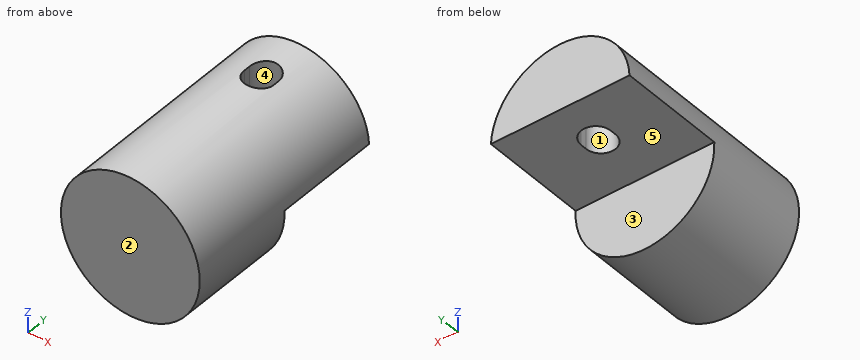
```python
from build123d import *

# Parameters (mm, degrees)
SKETCH1_R               = 9.75
BOSS_EXTRUDE1_DEPTH     = 30
CUT_EXTRUDE1_DEPTH      = 0.5
CUT_EXTRUDE1_DEPTH_BACK = 30
SKETCH3_W               = 19.5
SKETCH3_H               = 15
CUT_EXTRUDE2_DEPTH      = 30


with BuildPart() as part:
    # Sketch1 → Boss-Extrude1 (new body)
    with BuildSketch(Plane(origin=(0, 0, 0), x_dir=(1, 0, 0), z_dir=(0, 1, 0))):
        with Locations(Location((0, 0, 0), (0, 0, 270))):
            Circle(SKETCH1_R)
    extrude(amount=BOSS_EXTRUDE1_DEPTH)

    # Sketch3 → Cut-Extrude1 (cut, two sides: drawn at the far end of the back side and taken through both)
    with BuildSketch(Plane.XY.offset(-CUT_EXTRUDE1_DEPTH_BACK)):
        with Locations((0, 22.5)):
            Rectangle(SKETCH3_W, SKETCH3_H)
    extrude(amount=CUT_EXTRUDE1_DEPTH + CUT_EXTRUDE1_DEPTH_BACK, mode=Mode.SUBTRACT)

    # Sketch4 → Cut-Extrude2 (cut)
    with BuildSketch(Plane(origin=(0, 0, 0.5), x_dir=(-1, 0, 0), z_dir=(0, 0, -1))):
        with BuildLine():
            Line((2.06, 23.683843632), (2.06, 22.803843632))
            ThreePointArc((2.06, 22.803843632), (0, 20.743843632), (-2.06, 22.803843632))
            Line((-2.06, 22.803843632), (-2.06, 23.683843632))
            ThreePointArc((-2.06, 23.683843632), (0, 25.743843632), (2.06, 23.683843632))
        make_face()
    extrude(amount=-CUT_EXTRUDE2_DEPTH, mode=Mode.SUBTRACT)


solid = part.part
```
The listing builds one solid part. Answer for the finished solid, in the listing's coordinates (mm). Face numbers are marked on the shaded views. A direction names the side the tool comes from. Coordinates: 2 decimals unless noted, no trailing zeros. Write each loop counter-clockwise with the first axis right and the second up, starting at its lowest first coordinate (ties: lowest second). Pieces come first, ordered by that corner, then holes. Notation, with made-up numbers: (60, -37) -> (101, -37) arc R21 ccw to (101, -18) -> close; hole circle Ø4 at (66.5, 23). An arc over 180 degrees is marked (long way). Write each question's results on one line, items separated by ' | '. Start each with the question number.
1) A tool of negligible diameter and unlimited length cuts with its end or side. For the marked faces 1 and 2, from which of +Z, -Z, +X, -X, +Y, -Y can it reach the whole face along a straight path? Write none if from no direction.
2) A cutting plane is placed at A-A (x = 0). Determine the outline of the cut face in (y, z).
3) A cutting plane is placed at B-B (z = 3.75). Determine the outline of the cut face in (x, y).
4) For a pull along Y with two mould halves and no side action, classify the marked faces 3, 4 and 5 as +Y half, -Y half, draft (parallel to the pull), parting line (faces both ways), or undercut.
5) Straight lines are drawn through the part: probe 1 along X at (y, z) = (12, 0.25); probe 2 along Y at (x, z) = (-4.75, -2.75); probe 3 along Y at (x, z) = (0, 3). For each, find the intervals that lie inside material, in ascending order.
6) A cutting plane is placed at D-D (y = 5.5). Determine the outline of the cut face in (x, z), then the cut area to 3 significant figures.
7) A cutting plane is placed at C-C (y = 25). Determine the outline of the cut face in (x, z), then the cut area to 3 significant figures.
8) Flat-ended cylindrical pins translate along their axes: pin 1 Ø5 at (y, z) = (15, 6.5) entering from +X; pin 2 Ø10 at (y, z) = (20, 2) entering from -X; pin 3 Ø1 at (y, z) = (23, 5.5) entering from -X. Find the tip coordinate at first contact, or state that the pin passes through.
Values follow:
1) face 1: +Z, -Z | face 2: +Z, -Z, +X, -X, -Y
2) outline: (0, -9.75) -> (15, -9.75) -> (15, 0.5) -> (20.74, 0.5) -> (20.74, 9.75) -> (0, 9.75) -> close; (25.74, 0.5) -> (30, 0.5) -> (30, 9.75) -> (25.74, 9.75) -> close
3) outline: (-9, 0) -> (9, 0) -> (9, 30) -> (-9, 30) -> close; hole (-2.06, 22.8) arc R2.06 ccw to (2.06, 22.8) -> (2.06, 23.68) arc R2.06 ccw to (-2.06, 23.68) -> close
4) face 3: +Y half | face 4: undercut | face 5: draft
5) probe 1: -9.75 to 9.75 | probe 2: 0 to 15 | probe 3: 0 to 20.74, 25.74 to 30
6) outline: circle Ø19.5 at (0, 0) | area: 299 mm²
7) outline: (-9.74, 0.5) -> (-1.58, 0.5) -> (-1.58, 9.62) arc R9.75 ccw to start; (1.58, 0.5) -> (9.74, 0.5) arc R9.75 ccw to (1.58, 9.62) -> close | area: 110 mm²
8) pin 1: x = 8.89 | pin 2: x = -9.74 | pin 3: x = -8.37
